For this review, take the finished solid that the model builds, in its own axes (mm). A direction names the side the tool comes from. Coordinates: 2 decimals unless noted, no trailing zeros. Loops run counter-clockwise (first coordinate to the right, second up) from the corner with the lowest first, then second, coordinate; pieces in that order, holes last.
```python
from build123d import *

# Parameters (mm, degrees)
BOSS_EXTRUDE1_DEPTH = 25
SKETCH4_R           = 4
SKETCH4_R_2         = 1.5
CUT_EXTRUDE3_DEPTH  = 2
SKETCH5_R           = 1.5
SKETCH5_R_2         = 4
CUT_EXTRUDE4_DEPTH  = 2
SKETCH6_R           = 4
SKETCH6_R_2         = 1.5
CUT_EXTRUDE5_DEPTH  = 2
FILLET2_R           = 2


with BuildPart() as part:
    # Sketch1 → Boss-Extrude1 (new body)
    with BuildSketch(Plane.XY):
        Polygon((27.999082786, 67), (25.999082786, 67), (25.999082786, 2), (-26.000917214, 2), (-29.000917214, 67), (-30.998790434, 66.907790467), (-27.910738566, 0), (-26.000917214, 0), (27.999082786, 0), align=None)
    extrude(amount=-BOSS_EXTRUDE1_DEPTH)

    # Sketch4 → Cut-Extrude3 (cut)
    with BuildSketch(Plane(origin=(-27.851410119, -1.285449698, 0), x_dir=(0, 0, 1), z_dir=(-0.99893661, -0.046104767, 0))):
        with BuildLine():
            Line((0, 68.265833379), (-12.5, 68.265833379))
            ThreePointArc((-12.5, 68.265833379), (-3.661165235, 64.604668144), (0, 55.765833379))
            Line((0, 55.765833379), (0, 68.265833379))
        make_face()
        with BuildLine():
            Line((-25, 68.265833379), (-25, 55.765833379))
            ThreePointArc((-25, 55.765833379), (-21.338834765, 64.604668144), (-12.5, 68.265833379))
            Line((-12.5, 68.265833379), (-25, 68.265833379))
        make_face()
        with Locations((-12.5, 53.286818087)):
            Circle(SKETCH4_R)
        with Locations((-12.5, 34.786818087)):
            Circle(SKETCH4_R_2)
        with Locations((-12.5, 17.786818087)):
            Circle(SKETCH4_R_2)
        with Locations((-12.5, 46.286818087)):
            Circle(SKETCH4_R_2)
        with Locations((-19.5, 53.286818087)):
            Circle(SKETCH4_R_2)
        with Locations((-12.5, 60.286818087)):
            Circle(SKETCH4_R_2)
        with Locations((-5.5, 53.286818087)):
            Circle(SKETCH4_R_2)
    extrude(amount=-CUT_EXTRUDE3_DEPTH, mode=Mode.SUBTRACT)

    # Sketch5 → Cut-Extrude4 (cut)
    with BuildSketch(Plane(origin=(27.999082786, 0, 0), x_dir=(0, 0, -1), z_dir=(1, 0, 0))):
        with BuildLine():
            Line((0, 67), (0, 54.5))
            ThreePointArc((0, 54.5), (3.661165235, 63.338834765), (12.5, 67))
            Line((12.5, 67), (0, 67))
        make_face()
        with BuildLine():
            Line((25, 67), (12.5, 67))
            ThreePointArc((12.5, 67), (21.338834765, 63.338834765), (25, 54.5))
            Line((25, 54.5), (25, 67))
        make_face()
        with Locations((12.5, 59)):
            Circle(SKETCH5_R)
        with Locations((19.5, 52)):
            Circle(SKETCH5_R)
        with Locations((12.5, 45)):
            Circle(SKETCH5_R)
        with Locations((5.5, 52)):
            Circle(SKETCH5_R)
        with Locations((12.5, 33.5)):
            Circle(SKETCH5_R)
        with Locations((12.5, 16.5)):
            Circle(SKETCH5_R)
        with Locations((12.5, 52)):
            Circle(SKETCH5_R_2)
    extrude(amount=-CUT_EXTRUDE4_DEPTH, mode=Mode.SUBTRACT)

    # Sketch6 → Cut-Extrude5 (cut)
    with BuildSketch(Plane(origin=(0, 2, 0), x_dir=(1, 0, 0), z_dir=(0, 1, 0))):
        with Locations((-0.000917214, 12.5)):
            Circle(SKETCH6_R)
        with Locations((-7.000917214, 12.5)):
            Circle(SKETCH6_R_2)
        with Locations((-0.000917214, 19.5)):
            Circle(SKETCH6_R_2)
        with Locations((6.999082786, 12.5)):
            Circle(SKETCH6_R_2)
        with Locations((-0.000917214, 5.5)):
            Circle(SKETCH6_R_2)
        with Locations((18.499082786, 12.5)):
            Circle(SKETCH6_R_2)
        with Locations((-18.500917214, 12.5)):
            Circle(SKETCH6_R_2)
    extrude(amount=-CUT_EXTRUDE5_DEPTH, mode=Mode.SUBTRACT)

    # Fillet2
    fillet2_edges = [part.edges().sort_by_distance(p)[0] for p in [
        (-27.910738566, 0, -12.5),
        (-26.000917214, 2, -12.5),
        (25.999082786, 2, -12.5),
        (27.999082786, 0, -12.5),
    ]]
    fillet(fillet2_edges, radius=FILLET2_R)


solid = part.part
```
Q1. Machinability: for faces 4 (the face through (1, 1, 0)), 5 (the face through (27.013, 50.536, -5.175)), 6 (the face through (25.43, 2.6, -12.68)), which of the approach directions +Z, -Z, +X, -X, +Y, -Y give a long, thin tool a straight path to every point of the face, cutting with its end or side? Answer none if there is none.
Q2. Consider section A-A (z = -5.5). State the section outline as (x, y) points.
Q3. Wall thickness on probe 1 along Y at (x, z) = (2.5, -20); probe 2 along X at (y, z) = (54.5, -16); probe 3 along X at (y, z) = (0.65, -12.5): over which ranges is each line inside the solid? List them lowest first.
Q4. Consider section D-D (z = -9.75). State the section outline as (x, y) points, then the cut area to 3 significant figures.
Q5. The part is to be moulded in two halves that separate along Z. For faces 1 (the face through (-27.37, 0.54, -12.68)), 2 (the face through (1, 1, -25)), 3 (the face through (-5.57, 1.01, -12.95)), say which applies: +Z half, -Z half, draft (parallel to the pull), parting line (faces both ways), or undercut.
Q6. For pin 1 Ø13 at (x, z) = (0, -12.5) entering from +Y; pin 2 Ø9 at (y, z) = (52, -12.5) entering from -X; pin 3 Ø3.5 at (y, z) = (52, -5.5) entering from -X, all flat-tipped, find the tip position at first contact; note any pin that passes through.
Q7. Consider section B-B (x = 19). State the section outline as (y, z) points.
Q8. Consider section C-C (y = 20). State the section outline as (x, z) points.
Model answer:
1. face 4: +Z, +X, -X, +Y, -Y
1. face 5: +X
1. face 6: +Z, -Z, +Y
2. outline: (-30.9, 64.77) - (-30.38, 53.44) - (-28.38, 53.54) - (-28.9, 64.86) - close; (-30.24, 50.45) - (-28, 1.91) arc R2 ccw to (-26, 0) - (-1.5, 0) - (-1.5, 2) - (-24.09, 2) arc R2 cw to (-26.09, 3.91) - (-28.24, 50.54) - close; (1.5, 0) - (26, 0) arc R2 ccw to (28, 2) - (28, 50.5) - (26, 50.5) - (26, 4) arc R2 cw to (24, 2) - (1.5, 2) - close; (26, 53.5) - (28, 53.5) - (28, 64.86) - (26, 64.86) - close
3. probe 1: y = 0 to 2
3. probe 2: x = -30.43 to -28.42, 26 to 28
3. probe 3: x = -27.48 to -20, -17 to -8.5, -5.5 to -4, 4 to 5.5, 8.5 to 17, 20 to 27.47
4. outline: (-30.98, 66.6) - (-30.44, 54.85) - (-28.44, 54.94) - (-28.99, 66.69) - close; (-30.17, 49.04) - (-28, 1.91) arc R2 ccw to (-26, 0) - (-2.91, 0) - (-2.91, 2) - (-24.09, 2) arc R2 cw to (-26.09, 3.91) - (-28.18, 49.14) - close; (2.9, 0) - (26, 0) arc R2 ccw to (28, 2) - (28, 49.1) - (26, 49.1) - (26, 4) arc R2 cw to (24, 2) - (2.9, 2) - close; (26, 54.9) - (28, 54.9) - (28, 66.69) - (26, 66.69) - close
4. area: 336 mm2
5. face 1: draft
5. face 2: -Z half
5. face 3: undercut
6. pin 1: stops at y = 2
6. pin 2: stops at x = -30.52
6. pin 3: stops at x = -30.39
7. outline: (0, -25) - (2, -25) - (2, -13.91) - (0, -13.91) - close; (0, -11.09) - (2, -11.09) - (2, 0) - (0, 0) - close
8. outline: (-28.83, -25) - (-26.83, -25) - (-26.83, 0) - (-28.83, 0) - close; (26, -25) - (28, -25) - (28, 0) - (26, 0) - close
